The listing builds one solid part. Answer for the finished solid, in the listing's coordinates (mm). A direction names the side the tool comes from. Give positions to 0.01 mm unless a question says otherwise; leave off trailing zeros. Loops run counter-clockwise (first coordinate to the right, second up) from the corner with the lowest first, then second, coordinate; pieces in that order, holes last.
Item 1: Section D-D, the plane y = 13 is taken. Give the vertices of the cut face in (x, z), and give its area (3 significant figures).
Item 2: A tool of negligible diameter and unlimited length cuts with its end or side. For faces 1 (the face through (13, 0, 0)), 2 (the face through (0.04, 0, -0.14)), from which of +Z, -Z, +X, -X, +Y, -Y can it reach the whole face along a straight path? Write none if from no direction.
Item 3: Each of these flat-tipped pins is pushed along its axis until it touches: pin 1 Ø6 at (x, y) = (14.5, 2.5) entering from -Z; pin 2 Ø2.5 at (y, z) = (7.27, 0) entering from +X; pin 3 Ø9 at (x, z) = (15, -0.5) entering from +Y; pin 4 Ø1.5 at (y, z) = (8, 1) entering from +X. Where does it stop, or does it pass through?
Item 4: Section C-C, the plane z = -6 is taken. Give the vertices of the cut face in (x, y), and give its area (3 significant figures).
Item 5: Section A-A, the plane y = 7.27 is taken. Give the vertices of the cut face in (x, z), and give its area (3 significant figures).
Item 6: Consider line 1 along Z through (x, y) = (-0.3, 7.27); line 2 along X through (y, z) = (4.5, -4.75). Determine where each line is inside the solid, lowest interval first.
Item 7: Section B-B, the plane x = 10.8 is taken. Give the vertices of the cut face in (y, z), and give its area (3 significant figures).
Item 8: The mould has two halves that part along X. Classify faces 3 (the face through (-0.394, 8.784, 0.477)), 4 (the face through (8.863, -0.394, -0.43)), 5 (the face through (0, 16, 0)): pulls with the +X half, pulls with the -X half, needs draft (parallel to the pull), parting line crosses it, or undercut.
from build123d import *

# Parameters (mm, degrees)
BASE_FLANGE1_DEPTH      = 10
BASE_FLANGE1_DEPTH_BACK = 10
SKETCH2_R               = 1.5875
CUT_EXTRUDE1_DEPTH      = 38.416573868
SKETCH3_R               = 1.984375
CUT_EXTRUDE2_DEPTH      = 10
FILLET1_R               = 3


# Sheet-metal steps are written as plain solids
with BuildPart() as part:
    # Sketch1 → Base-Flange1 (new, two sides: drawn at the far end of the back side and taken through both)
    with BuildSketch(Plane.XY.offset(-BASE_FLANGE1_DEPTH_BACK)):
        with BuildLine():
            Line((0, 30), (0, 2))
            ThreePointArc((0, 2), (0.585786438, 0.585786438), (2, 0))
            Line((2, 0), (20, 0))
            Line((20, 0), (20, -0.8))
            Line((20, -0.8), (2, -0.8))
            ThreePointArc((2, -0.8), (0.020101013, 0.020101013), (-0.8, 2))
            Line((-0.8, 2), (-0.8, 30))
            Line((-0.8, 30), (0, 30))
        make_face()
    extrude(amount=BASE_FLANGE1_DEPTH + BASE_FLANGE1_DEPTH_BACK)

    # Sketch2 → Cut-Extrude1 (cut, through all)
    with BuildSketch(Plane(origin=(0, 0, 0), x_dir=(0, 0, -1), z_dir=(1, 0, 0))):
        with Locations(Location((0, 7.27, 0), (0, 0, 90))):
            Circle(SKETCH2_R)
    extrude(amount=-CUT_EXTRUDE1_DEPTH, mode=Mode.SUBTRACT)

    # Sketch3 → Cut-Extrude2 (cut)
    with BuildSketch(Plane(origin=(0, 0, 0), x_dir=(1, 0, 0), z_dir=(0, 1, 0))):
        with Locations(Location((10.8, 0, 0), (0, 0, 270))):
            Circle(SKETCH3_R)
    extrude(amount=-CUT_EXTRUDE2_DEPTH, mode=Mode.SUBTRACT)

    # Fillet1
    fillet1_edges = [part.edges().sort_by_distance(p)[0] for p in [
        (-0.4, 30, 10),
        (-0.4, 30, -10),
    ]]
    fillet(fillet1_edges, radius=FILLET1_R)


solid = part.part
Worked answers:
1. outline: (-0.8, -10) - (0, -10) - (0, 10) - (-0.8, 10) - close
1. area: 16.0 mm2
2. face 1: +Z, -Z, +X, +Y
2. face 2: +Z, -Z, -X, -Y
3. pin 1: stops at z = -10
3. pin 2: passes through
3. pin 3: stops at y = 0
3. pin 4: stops at x = 0
4. outline: (-0.8, 2) arc R2.8 ccw to (2, -0.8) - (20, -0.8) - (20, 0) - (2, 0) arc R2 cw to (0, 2) - (0, 30) - (-0.8, 30) - close
4. area: 39.8 mm2
5. outline: (-0.8, -10) - (0, -10) - (0, -1.59) - (-0.8, -1.59) - close; (-0.8, 1.59) - (0, 1.59) - (0, 10) - (-0.8, 10) - close
5. area: 13.5 mm2
6. line 1: z = -10 to -1.59, 1.59 to 10
6. line 2: x = -0.8 to 0
7. outline: (-0.8, -10) - (0, -10) - (0, -1.98) - (-0.8, -1.98) - close; (-0.8, 1.98) - (0, 1.98) - (0, 10) - (-0.8, 10) - close
7. area: 12.8 mm2
8. face 3: needs draft
8. face 4: undercut
8. face 5: pulls with the +X half
